Could you check a few things on this model? Use its own coordinates, in mm. Coordinates: 2 decimals unless noted, no trailing zeros. Loops run counter-clockwise (first coordinate to the right, second up) from the corner with the lowest first, then second, coordinate; pieces in that order, holes last.
from build123d import *

# Parameters (mm, degrees)
F1_DEPTH = 5
F2_R     = 10
F3_R     = 10
F4_R     = 2.5
F5_DEPTH = 25
F6_R     = 2.5
F7_DEPTH = 25
F9_DEPTH = 25
F10_R    = 5


with BuildPart() as f1:
    # F0 (on Front) → F1 (new body)
    with BuildSketch(Plane.XZ):
        with BuildLine():
            Line((-150, 0), (0, 0))
            Line((0, 0), (150, 0))
            Line((150, 0), (150, 40))
            Line((150, 40), (50.331140256, 60))
            ThreePointArc((50.331140256, 60), (25.289442854, 63.7469311095), (0, 65))
            ThreePointArc((0, 65), (-25.289442854, 63.7469311095), (-50.331140256, 60))
            Line((-50.331140256, 60), (-150, 40))
            Line((-150, 40), (-150, 0))
        make_face()
    extrude(amount=F1_DEPTH)

    # F2
    f2_edges = [f1.edges().sort_by_distance(p)[0] for p in [
        (150, -2.5, 40),
        (-150, -2.5, 40),
    ]]
    fillet(f2_edges, radius=F2_R)

    # F3
    f3_edges = [f1.edges().sort_by_distance(p)[0] for p in [
        (-150, -2.5, 0),
        (150, -2.5, 0),
    ]]
    fillet(f3_edges, radius=F3_R)

    # F4 (on face) → F5 (cut)
    with BuildSketch(Plane.XZ.offset(5)):
        with Locations((-50, 20)):
            Circle(F4_R)
        with Locations((50, 20)):
            Circle(F4_R)
        with Locations((0, 20)):
            Circle(F4_R)
    extrude(amount=-F5_DEPTH, mode=Mode.SUBTRACT)

    # F6 (on face) → F7 (cut)
    with BuildSketch(Plane.XZ.offset(5)):
        with Locations((-100, 12)):
            Circle(F6_R)
        with Locations((100, 12)):
            Circle(F6_R)
        with Locations((50, 20)):
            Circle(F6_R)
    extrude(amount=-F7_DEPTH, mode=Mode.SUBTRACT)

    # F8 (on face) → F9 (cut)
    with BuildSketch(Plane.XZ.offset(5)):
        with BuildLine():
            Line((-141.9674253139, 76.700784266), (-141.9674253139, 41.6118524295))
            Line((-141.9674253139, 41.6118524295), (-50.331140256, 60))
            ThreePointArc((-50.331140256, 60), (0, 65), (50.331140256, 60))
            Line((50.331140256, 60), (141.9674253139, 41.6118524295))
            Line((141.9674253139, 41.6118524295), (141.9674253139, 76.700784266))
            Line((141.9674253139, 76.700784266), (-141.9674253139, 76.700784266))
        make_face()
        with BuildLine():
            Line((-50.331140256, 60), (-141.9674253139, 41.6118524295))
            ThreePointArc((-141.9674253139, 41.6118524295), (0, 32.0253701889), (141.9674253139, 41.6118524295))
            Line((141.9674253139, 41.6118524295), (50.331140256, 60))
            ThreePointArc((50.331140256, 60), (0, 65), (-50.331140256, 60))
        make_face()
    extrude(amount=-F9_DEPTH, mode=Mode.SUBTRACT)

    # F10
    f10_edges = [f1.edges().sort_by_distance(p)[0] for p in [
        (-141.967425, -2.5, 41.611852),
        (141.967425, -2.5, 41.611852),
    ]]
    fillet(f10_edges, radius=F10_R)


solid = f1.part
(1) Imagine slicing it at B-B, the plane z = 20. Write out the boundary of the cut face in (x, y).
Answers:
outline: (-150, -5) - (-52.5, -5) - (-52.5, 0) - (-150, 0) - close; (-47.5, -5) - (-2.5, -5) - (-2.5, 0) - (-47.5, 0) - close; (2.5, -5) - (47.5, -5) - (47.5, 0) - (2.5, 0) - close; (52.5, -5) - (150, -5) - (150, 0) - (52.5, 0) - close
(2) For pin 1 (1 mm diameter, centred on x = -6, y = -4.5, fed in from +Z), with a flat end and sliding along its axis, tell me the tip position at first contact or that it passes through.
Answers:
pin 1: stops at z = 32.05
(3) Imagine slicing it at A-A, the plane x = 0. Write out the boundary of the cut face in (y, z), and give its area (3 significant figures).
Answers:
outline: (-5, 0) - (0, 0) - (0, 17.5) - (-5, 17.5) - close; (-5, 22.5) - (0, 22.5) - (0, 32.03) - (-5, 32.03) - close
area: 135 mm2
(4) We'd pull the mould along Z, two halves only. Please class faces 1 (the face through (148.21, -2.54, 37.52)), 2 (the face through (-0.33, -2.54, 22.48)), 3 (the face through (-2, -2, 0)), 4 (the face through (-2, -5, 16)): +Z half, -Z half, draft (parallel to the pull), parting line (faces both ways), or undercut.
Answers:
face 1: +Z half
face 2: undercut
face 3: -Z half
face 4: draft
(5) I need wall thicknesses on probe 1 along Z at (x, y) = (0, -1.3); probe 2 along X at (y, z) = (-3.55, 11); probe 3 along X at (y, z) = (-4.3, 32). Which ranges of each line are inside material? Lowest first, please.
Answers:
probe 1: z = 0 to 17.5, 22.5 to 32.03
probe 2: x = -150 to -102.29, -97.71 to 97.71, 102.29 to 150
probe 3: x = -150 to 150
(6) Imagine slicing it at D-D, the plane x = 100. Write out the boundary of the cut face in (y, z), and give its area (3 significant figures).
Answers:
outline: (-5, 0) - (0, 0) - (0, 9.5) - (-5, 9.5) - close; (-5, 14.5) - (0, 14.5) - (0, 36.77) - (-5, 36.77) - close
area: 159 mm2
(7) Imagine slicing it at C-C, the plane y = -3. State how many separate pieces and enclosed holes the cut face has, and give its area (3 significant figures).
Answers:
separate pieces: 1
enclosed holes: 5
area: 10,500 mm2
